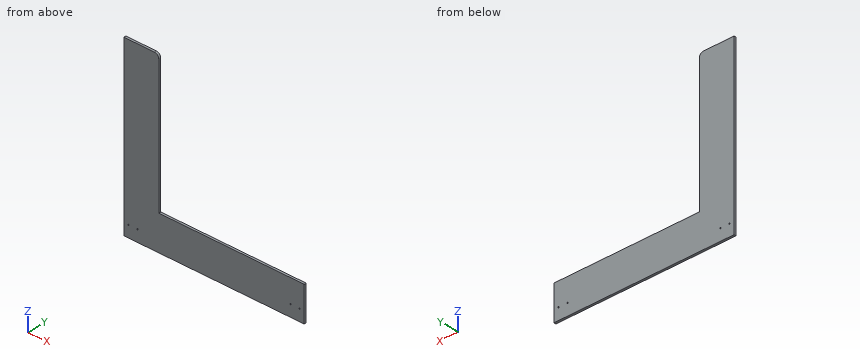
```python
from build123d import *

# Parameters (mm, degrees)
F1_DEPTH = 19.05
F2_R     = 6.35
F4_D     = 11.1252


with BuildPart() as f1:
    # F0 (on Front) → F1 (new body)
    with BuildSketch(Plane.XZ):
        with BuildLine():
            Line((1371.6, 304.8), (304.8, 304.8))
            Line((304.8, 304.8), (304.8, 1485.9))
            ThreePointArc((304.8, 1485.9), (293.640768, 1512.840768), (266.7, 1524))
            Line((266.7, 1524), (0, 1524))
            Line((0, 1524), (0, 0))
            Line((0, 0), (1574.8, 0))
            Line((1574.8, 0), (1574.8, 304.8))
            Line((1574.8, 304.8), (1371.6, 304.8))
        make_face()
    extrude(amount=F1_DEPTH)

    # F2
    f2_edges = [f1.edges().sort_by_distance(p)[0] for p in [
        (1574.8, -9.525, 304.8),
    ]]
    fillet(f2_edges, radius=F2_R)

    # F4 (through all)
    with Locations(Plane.XZ.offset(19.05)):
        with Locations((1535.1252, 101.6), (1455.7502, 101.6), (119.0498, 101.6), (39.6748, 101.6)):
            Hole(F4_D / 2)


solid = f1.part
```
Could you check a few things on this model? Use its own coordinates, in mm. Give positions to 0.01 mm unless a question says otherwise; leave off trailing zeros. Write each loop counter-clockwise with the first axis right and the second up, starting at its lowest first coordinate (ties: lowest second). Pieces come first, ordered by that corner, then holes. Notation, with made-up numbers: (2.25, 4.5) - (55.25, 4.5) arc R19 ccw to (55.25, 18.5) - close; hole circle Ø8 at (24.5, 70.5). An arc over 180 degrees is marked (long way). One line per item, written item: value. Start each with the question number.
Item 1: Imagine slicing it at B-B, the plane z = 438.5. List the corners of the cut face in (x, y) for me, and give its area (3 significant figures).
Item 2: Imagine slicing it at A-A, the plane y = -3. List the corners of the cut face in (x, z) for me.
Item 3: Imagine slicing it at C-C, the plane x = 1276. List the corners of the cut face in (y, z) for me, and give its area (3 significant figures).
Item 4: Please list where these lines run through material, in increasing order: line 1 (X direction, y = -8.5, z = 1039); line 2 (Z direction, x = 271, y = -17.5). Write a range as from..to.
Item 5: I'm going to push flat-ended pins straight in: pin 1 (3 mm diameter, centred on y = -3.5, z = 559.5, fed in from +X); pin 2 (4 mm diameter, centred on x = 1091.5, y = -10.5, fed in from +Z). Where does each tip first touch, or does it pass through?
Geometry says:
1. outline: (0, -19.05) - (304.8, -19.05) - (304.8, 0) - (0, 0) - close
1. area: 5,810 mm^2
2. outline: (0, 0) - (1574.8, 0) - (1574.8, 298.45) arc R6.35 ccw to (1568.45, 304.8) - (304.8, 304.8) - (304.8, 1485.9) arc R38.1 ccw to (266.7, 1524) - (0, 1524) - close; hole circle Ø11.13 at (39.67, 101.6); hole circle Ø11.13 at (119.05, 101.6); hole circle Ø11.13 at (1455.75, 101.6); hole circle Ø11.13 at (1535.13, 101.6)
3. outline: (-19.05, 0) - (0, 0) - (0, 304.8) - (-19.05, 304.8) - close
3. area: 5,810 mm^2
4. line 1: 0..304.8
4. line 2: 0..1523.76
5. pin 1: x = 304.8
5. pin 2: z = 304.8
